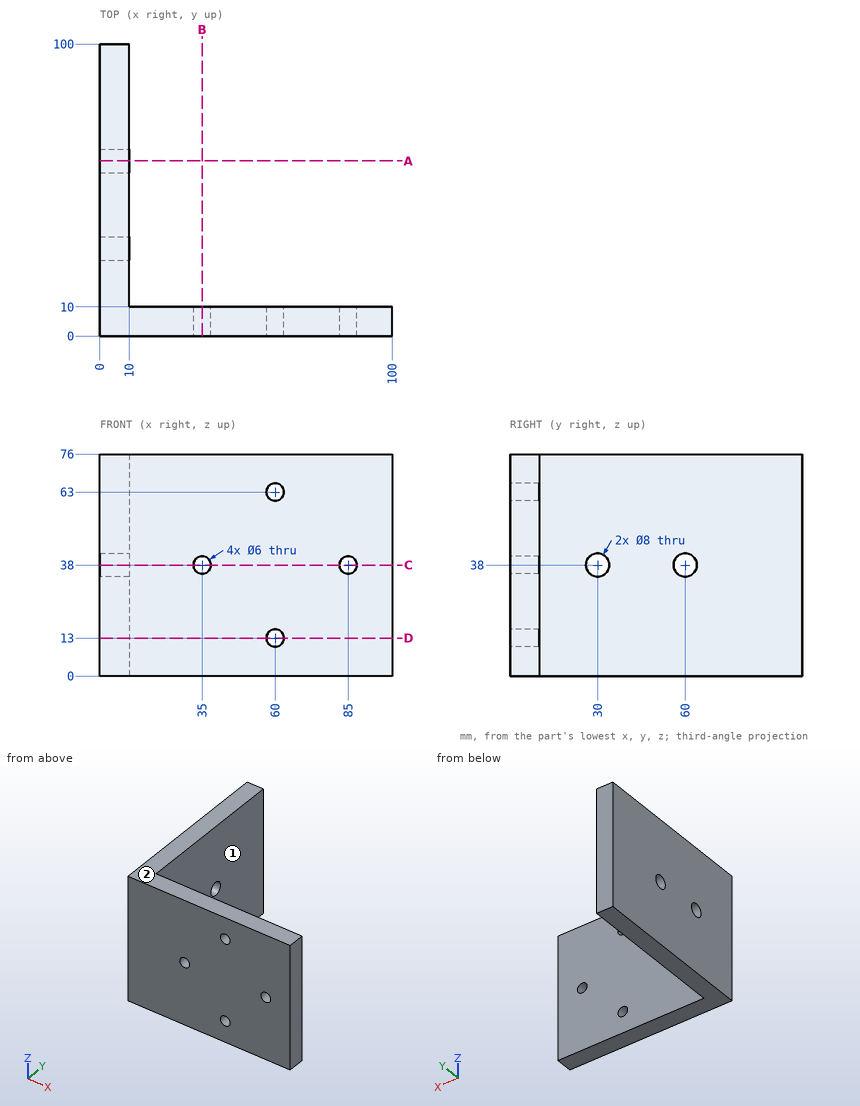
Geometry check sheet. Reference: drawing and pictorial views, mm from the part's lowest x, y, z. A direction names the side the tool comes from. Round coordinates to 2 decimals unless told otherwise and drop trailing zeros. Loops run counter-clockwise (first coordinate to the right, second up) from the corner with the lowest first, then second, coordinate; pieces in that order, holes last. Notation, with made-up numbers: M -6.75,-39 L 1.25,-39 A27 ccw 1.25,-14 Z; hole C -15,70 d9. An arc over 180 degrees is marked long. Return JSON: item names as keys, results as strings. Group by question number.
(1) Set-up check for the marked faces 1 and 2: record each of +Z, -Z, +X, -X, +Y, -Y from which the full face is reachable in a straight line by a thin tool's end or side.
(2) Section check C-C, the plane z = 38. Enter the section's corners in (x, y).
(3) Scan lines: line 1 along X through (y, z) = (7, 38); line 2 along Y through (x, z) = (2, 38); line 3 along X through (y, z) = (6, 13). Record each from-to range of solid material in increasing order. Write a range as [from, to].
(4) Section check D-D, the plane z = 13. Enter the section's corners in (x, y), and give its area (3 significant figures).
(5) Go/stop test with flat-tipped pins: pin 1 (1.5 mm diameter, centred on y = 23, z = 9.5, fed in from +X); pin 2 (3.5 mm diameter, centred on x = 35, z = 38, fed in from +Y); pin 3 (7 mm diameter, centred on x = 85, z = 38, fed in from +Y). Record where each tip stops, or that it passes through.
(6) Section check A-A, the plane y = 60. Enter the section's corners in (x, z), and give its area (3 significant figures).
(7) Section check B-B, the plane x = 35. Enter the section's corners in (y, z).
Data:
{
 "1": {"face 1": "+Z, -Z, +X, +Y", "face 2": "+Z, +X, -X, +Y, -Y"},
 "2": {"outline": "M 0,0 L 32,0 L 32,10 L 10,10 L 10,26 L 0,26 Z; M 0,34 L 10,34 L 10,56 L 0,56 Z; M 0,64 L 10,64 L 10,100 L 0,100 Z; M 38,0 L 82,0 L 82,10 L 38,10 Z; M 88,0 L 100,0 L 100,10 L 88,10 Z"},
 "3": {"line 1": "[0, 32], [38, 82], [88, 100]", "line 2": "[0, 26], [34, 56], [64, 100]", "line 3": "[0, 57], [63, 100]"},
 "4": {"outline": "M 0,0 L 57,0 L 57,10 L 10,10 L 10,100 L 0,100 Z; M 63,0 L 100,0 L 100,10 L 63,10 Z", "area": "1,840 mm²"},
 "5": {"pin 1": "x = 10", "pin 2": "through", "pin 3": "y = 10"},
 "6": {"outline": "M 0,0 L 10,0 L 10,34 L 0,34 Z; M 0,42 L 10,42 L 10,76 L 0,76 Z", "area": "680 mm²"},
 "7": {"outline": "M 0,0 L 10,0 L 10,35 L 0,35 Z; M 0,41 L 10,41 L 10,76 L 0,76 Z"}
}
